For this review, use the dimensioned drawing (mm, ordinates from the lowest corner) and the shaded views. Coordinates: 2 decimals unless noted, no trailing zeros. Write each loop counter-clockwise with the first axis right and the second up, starting at its lowest first coordinate (ties: lowest second). Pieces come first, ordered by that corner, then holes. Notation, with made-up numbers: (-23.75, 6) - (33.25, 6) arc R13 cw to (33.25, 13) - close; hole circle Ø7 at (-6, 49). An arc over 180 degrees is marked (long way). One line per item, written item: value.
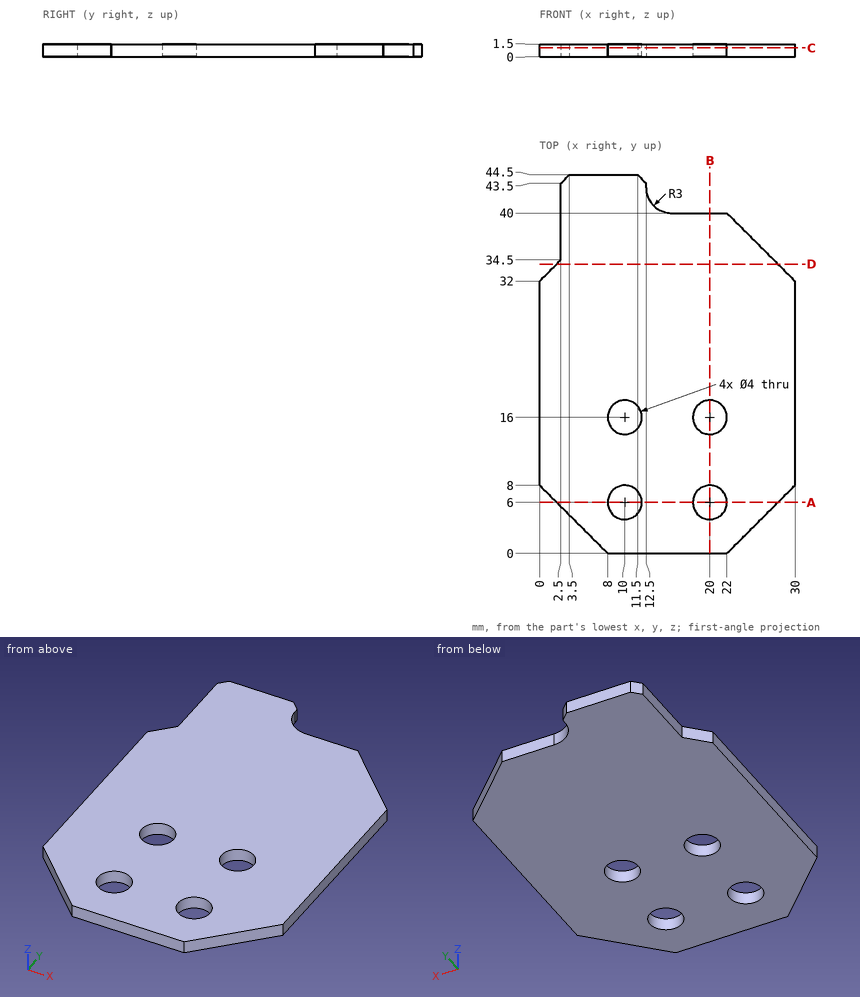
1. Consider section B-B, the plane x = 20. Write out the cut boundary in (y, z).
Answer block:
outline: (0, 0) - (4, 0) - (4, 1.5) - (0, 1.5) - close; (8, 0) - (14, 0) - (14, 1.5) - (8, 1.5) - close; (18, 0) - (40, 0) - (40, 1.5) - (18, 1.5) - close
2. Consider section A-A, the plane y = 6. Write out the cut boundary in (x, z), then the cut area to 3 significant figures.
Answer block:
outline: (2, 0) - (8, 0) - (8, 1.5) - (2, 1.5) - close; (12, 0) - (18, 0) - (18, 1.5) - (12, 1.5) - close; (22, 0) - (28, 0) - (28, 1.5) - (22, 1.5) - close
area: 27.0 mm^2
3. Consider section C-C, the plane z = 1.05. Write out the cut boundary in (x, y), then the cut area to 3 significant figures.
Answer block:
outline: (0, 8) - (8, 0) - (22, 0) - (30, 8) - (30, 32) - (22, 40) - (15.5, 40) arc R3 cw to (12.5, 43) - (12.5, 43.5) - (11.5, 44.5) - (3.5, 44.5) - (2.5, 43.5) - (2.5, 34.5) - (0, 32) - close; hole circle Ø4 at (10, 6); hole circle Ø4 at (10, 16); hole circle Ø4 at (20, 6); hole circle Ø4 at (20, 16)
area: 1,080 mm^2
4. Wall thickness on line 1 along Y through (x, z) = (10, 0.7); line 2 along Y through (x, z) = (20, 0.4); line 3 along Y through (x, z) = (5.5, 0.45): over which ranges is each line inside the solid? List them lowest first.
Answer block:
line 1: y = 0 to 4, 8 to 14, 18 to 44.5
line 2: y = 0 to 4, 8 to 14, 18 to 40
line 3: y = 2.5 to 44.5
5. Consider section D-D, the plane y = 34. Write out the cut boundary in (x, z), then the cut area to 3 significant figures.
Answer block:
outline: (2, 0) - (28, 0) - (28, 1.5) - (2, 1.5) - close
area: 39.0 mm^2
6. Insertion check: pin 1 Ø2.5 at (x, y) = (20, 6) entering from -Z. The pin has a flat end and moves straight along its axis. Give the tip position at first contact, or say it passes through.
Answer block:
pin 1: passes through
